Job drawing, mm, ordinate dimensions from the low corner. One solid piece. Give positions to 0.01 mm unless a question says otherwise; leave off trailing zeros. Loops run counter-clockwise (first coordinate to the right, second up) from the corner with the lowest first, then second, coordinate; pieces in that order, holes last. Notation, with made-up numbers: (3.5, 12) - (22.5, 12) arc R28 ccw to (22.5, 44) - close; hole circle Ø6 at (-31, -9). An arc over 180 degrees is marked (long way). Use a Markdown table: item, result.
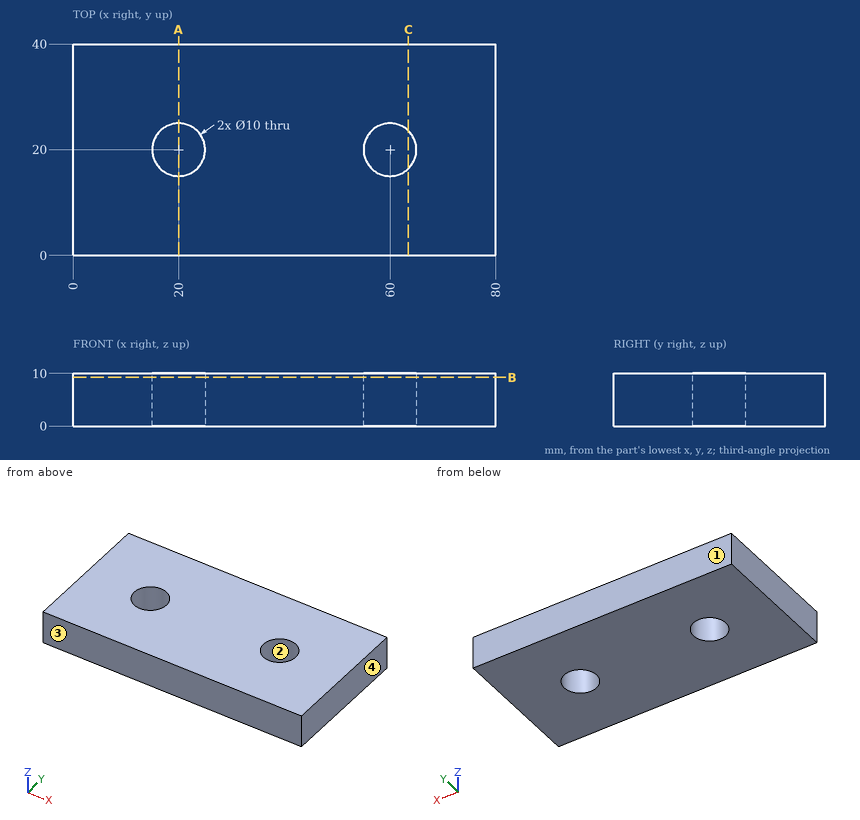
(1) Slice it at B-B, the plane z = 9.25. Write the cut outline in (x, y).
Computed:
| item | result |
|---|---|
| outline | (0, 0) - (80, 0) - (80, 40) - (0, 40) - close; hole circle Ø10 at (20, 20); hole circle Ø10 at (60, 20) |
(2) Slice it at A-A, the plane x = 20. Write the cut outline in (y, z).
Computed:
| item | result |
|---|---|
| outline | (0, 0) - (15, 0) - (15, 10) - (0, 10) - close; (25, 0) - (40, 0) - (40, 10) - (25, 10) - close |
(3) Drill centre lines: probe 1 along Y at (x, z) = (20, 6.75); probe 2 along X at (y, z) = (16.5, 1); probe 3 along Y at (x, z) = (18, 9). Where is each one in solid material? Low to high. Write a range as [from, to].
Computed:
| item | result |
|---|---|
| probe 1 | [0, 15], [25, 40] |
| probe 2 | [0, 16.43], [23.57, 56.43], [63.57, 80] |
| probe 3 | [0, 15.42], [24.58, 40] |
(4) Slice it at C-C, the plane x = 63.5. Write the cut outline in (y, z).
Computed:
| item | result |
|---|---|
| outline | (0, 0) - (16.43, 0) - (16.43, 10) - (0, 10) - close; (23.57, 0) - (40, 0) - (40, 10) - (23.57, 10) - close |
(5) Mould opens along Y. For the marked faces 1, 2, 3 and 4 say: pulls with the +Y half, pulls with the -Y half, needs draft (parallel to the pull), parting line crosses it, or undercut.
Computed:
| item | result |
|---|---|
| face 1 | pulls with the +Y half |
| face 2 | undercut |
| face 3 | pulls with the -Y half |
| face 4 | needs draft |
(6) Pin check, flat tip, straight feed: P1, Ø16, axis at x = 60, y = 20, coming from the -Z side. Stop position of the tip, or through.
Computed:
| item | result |
|---|---|
| P1 | z = 0 |
